Study the drawing (mm; zero at the part's minimum x, y, z) and answer. Round coordinates to 2 decimals unless told otherwise and drop trailing zeros. Loops run counter-clockwise (first coordinate to the right, second up) from the corner with the lowest first, then second, coordinate; pieces in that order, holes last. Notation, with made-up numbers: (77.25, 77) -> (117.25, 77) arc R23 ccw to (117.25, 87) -> close; hole circle Ø8 at (11.5, 65). An arc over 180 degrees is marked (long way). Use one line per item in the form item = value.
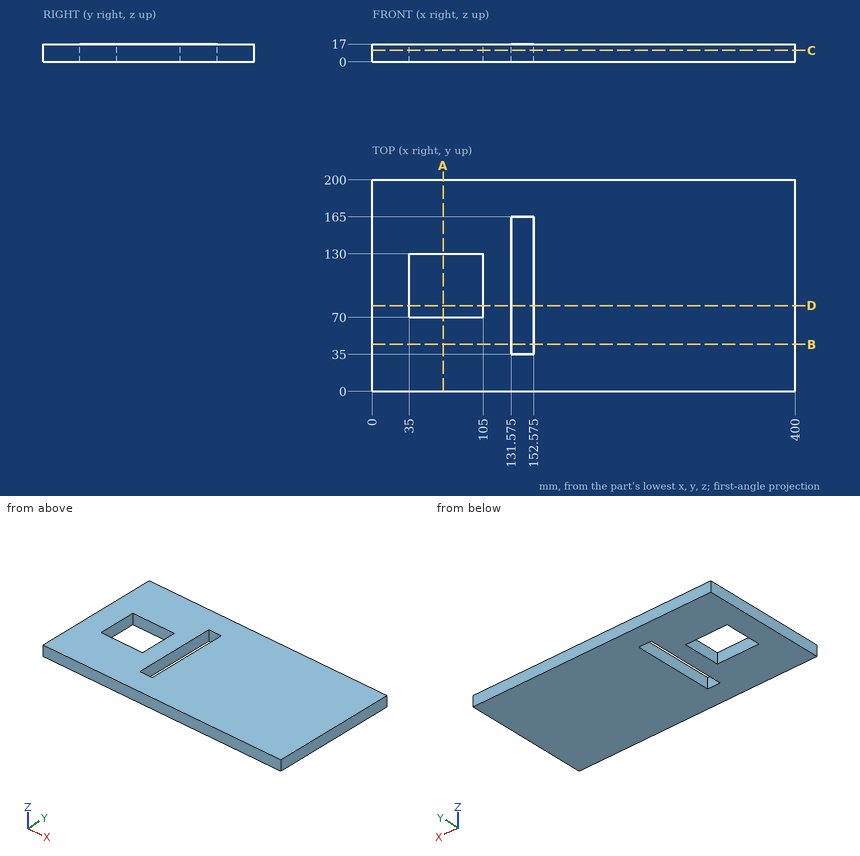
(1) Find section A-A, the plane x = 67. Write down the section's boundary in (y, z).
Completed:
outline = (0, 0) -> (70, 0) -> (70, 17) -> (0, 17) -> close; (130, 0) -> (200, 0) -> (200, 17) -> (130, 17) -> close
(2) Find section D-D, the plane y = 81. Write down the section's boundary in (x, z) (3 decimals), then the cut area to 3 significant figures.
Completed:
outline = (0, 0) -> (35, 0) -> (35, 17) -> (0, 17) -> close; (105, 0) -> (131.575, 0) -> (131.575, 17) -> (105, 17) -> close; (152.575, 0) -> (400, 0) -> (400, 17) -> (152.575, 17) -> close
area = 5,250 mm2
(3) Given P1, Ø8, axis at y = 76.5, z = 7, coming from the -X side, flat-ended and moving along its own axis, determine where the tip first touches the part or whether it passes through.
Completed:
P1 = 0
(4) Find section B-B, the plane y = 44.5. Write down the section's boundary in (x, z) (3 decimals), then the cut area to 3 significant figures.
Completed:
outline = (0, 0) -> (131.575, 0) -> (131.575, 17) -> (0, 17) -> close; (152.575, 0) -> (400, 0) -> (400, 17) -> (152.575, 17) -> close
area = 6,440 mm2
(5) Find section C-C, the plane z = 11. Write down the section's boundary in (x, y) (3 decimals), then the cut area to 3 significant figures.
Completed:
outline = (0, 0) -> (400, 0) -> (400, 200) -> (0, 200) -> close; hole (35, 70) -> (105, 70) -> (105, 130) -> (35, 130) -> close; hole (131.575, 35) -> (152.575, 35) -> (152.575, 165) -> (131.575, 165) -> close
area = 73,100 mm2
(6) Consider L1, parallel to Y at x = 70, z = 15.75; L2, parallel to X at y = 41, z = 5.25 (3 decimals). Determine where each line is inside the solid, lowest interval first.
Completed:
L1 = 0 to 70, 130 to 200
L2 = 0 to 131.575, 152.575 to 400
